The figure shows three views and two pictorial views of one solid part (mm, origin at its lowest corner). Answer the questions. Round coordinates to 2 decimals unless told otherwise and drop trailing zeros. Order: outer loops, then holes, each group sorted by start corner. A loop starts at its lowest first (then second) coordinate and runs counter-clockwise, first axis right, second up. Notation, with made-up numbers: M 62.25,7.25 L 108.25,7.25 A15 cw 108.25,25.25 Z; hole C 70.5,83 d9. An arc over 180 degrees is marked long. Return JSON: item names as keys, results as strings.
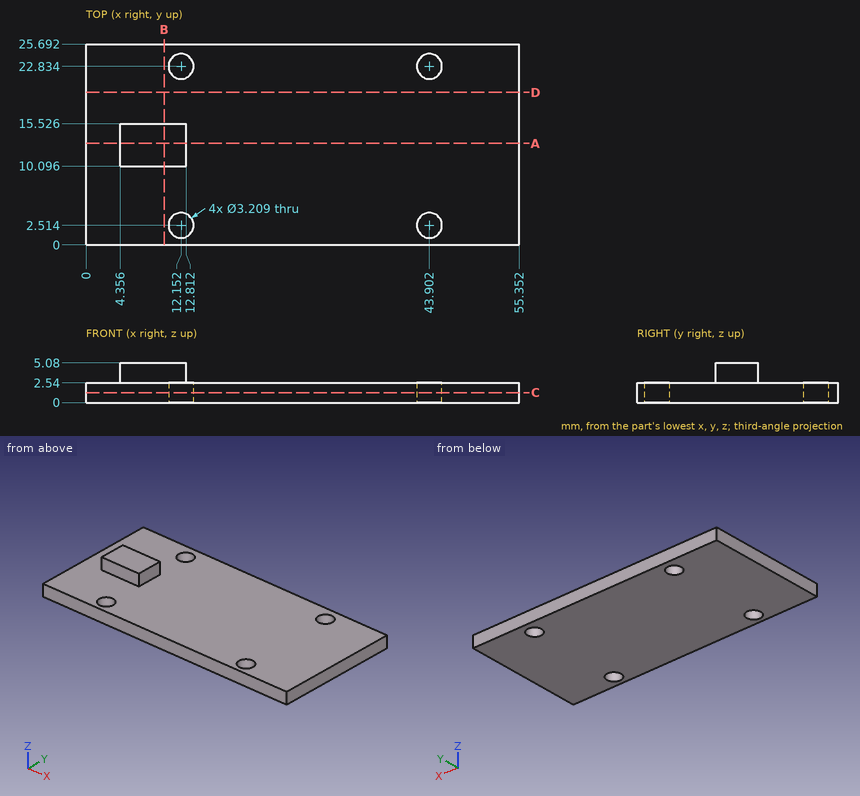
Item 1: Find section C-C (z = 1.3). Determine the outline of the cut face in (x, y) (1 decimal), plus the area to 3 significant figures.
Output:
{"outline": "M 0,0 L 55.4,0 L 55.4,25.7 L 0,25.7 Z; hole C 12.2,2.5 d3.2; hole C 12.2,22.8 d3.2; hole C 43.9,2.5 d3.2; hole C 43.9,22.8 d3.2", "area": "1,390 mm^2"}
Item 2: Find section A-A (y = 13). Determine the outline of the cut face in (x, z) (1 decimal), plus the area to 3 significant figures.
Output:
{"outline": "M 0,0 L 55.4,0 L 55.4,2.5 L 12.8,2.5 L 12.8,5.1 L 4.4,5.1 L 4.4,2.5 L 0,2.5 Z", "area": "162 mm^2"}
Item 3: Find section B-B (x = 10). Determine the outline of the cut face in (y, z) (1 decimal).
Output:
{"outline": "M 0,0 L 25.7,0 L 25.7,2.5 L 15.5,2.5 L 15.5,5.1 L 10.1,5.1 L 10.1,2.5 L 0,2.5 Z"}
Item 4: Find section D-D (y = 19.5). Determine the outline of the cut face in (x, z).
Output:
{"outline": "M 0,0 L 55.35,0 L 55.35,2.54 L 0,2.54 Z"}
Item 5: Consider line 1 along Z through (x, y) = (9, 7.5); line 2 along X through (y, z) = (14.75, 3.65) (1 decimal); line 3 along Y through (x, z) = (10, 3.9) (1 decimal). Determine where each line is inside the solid, lowest interval first. Write a range as [from, to].
Output:
{"line 1": "z = [0, 2.54]", "line 2": "x = [4.4, 12.8]", "line 3": "y = [10.1, 15.5]"}
Item 6: Each of these flat-tipped pins is pushed along its axis until it touches: pin 1 (4 mm diameter, centred on x = 43.9, y = 2.51, fed in from +Z); pin 2 (2 mm diameter, centred on y = 12.5, z = 4, fed in from -X); pin 3 (0.8 mm diameter, centred on x = 7.5, z = 3.5, fed in from +Y); pin 4 (3 mm diameter, centred on x = 12.15, y = 22.83, fed in from +Z). Where does it stop, or does it pass through?
Output:
{"pin 1": "stops at z = 2.54", "pin 2": "stops at x = 4.36", "pin 3": "stops at y = 15.53", "pin 4": "passes through"}
